The drawing under review shows one solid part. Ordinate dimensions are in mm from its lowest x, y, z. Coordinates: 2 decimals unless noted, no trailing zeros. Order: outer loops, then holes, each group sorted by start corner. A loop starts at its lowest first (then second) coordinate and runs counter-clockwise, first axis right, second up.
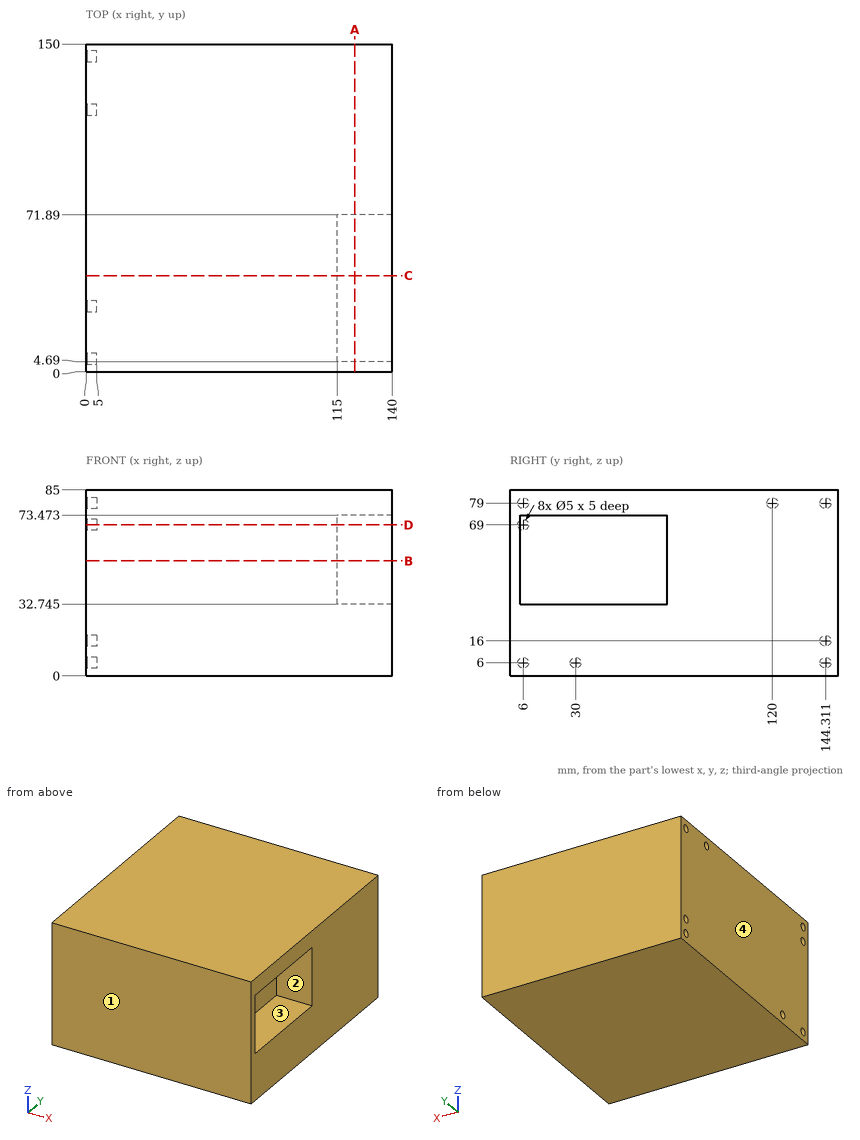
(1) Draft analysis for pull direction Y (two halves, no side actions). For the marked faces 1, 2, 3 and 4, state which applies: released by +Y, released by -Y, zero draft, split by the parting line, or undercut.
A:
face 1: released by -Y
face 2: undercut
face 3: undercut
face 4: zero draft
(2) We need section A-A, the plane x = 123. Write out the cut boundary in (y, z) (1 decimal).
A:
outline: (0, 0) - (150, 0) - (150, 85) - (0, 85) - close; hole (4.7, 32.7) - (71.9, 32.7) - (71.9, 73.5) - (4.7, 73.5) - close
(3) We need section D-D, the plane z = 69. Write out the cut boundary in (x, y), and give its area (3 significant figures).
A:
outline: (0, 0) - (140, 0) - (140, 4.69) - (115, 4.69) - (115, 71.89) - (140, 71.89) - (140, 150) - (0, 150) - (0, 8.5) - (5, 8.5) - (5, 3.5) - (0, 3.5) - close
area: 19,300 mm2
(4) We need section B-B, the plane z = 52.5. Write out the cut boundary in (x, y).
A:
outline: (0, 0) - (140, 0) - (140, 4.69) - (115, 4.69) - (115, 71.89) - (140, 71.89) - (140, 150) - (0, 150) - close
(5) We need section C-C, the plane y = 44. Write out the cut boundary in (x, z) (1 decimal).
A:
outline: (0, 0) - (140, 0) - (140, 32.7) - (115, 32.7) - (115, 73.5) - (140, 73.5) - (140, 85) - (0, 85) - close
(6) Wall thickness on probe 1 along Z at (x, y) = (3.9, 6); probe 2 along X at (y, z) = (55.5, 58): over which ranges is each line inside the solid? List them lowest first.
A:
probe 1: z = 0 to 3.5, 8.5 to 66.5, 71.5 to 76.5, 81.5 to 85
probe 2: x = 0 to 115
(7) For pin 1 Ø3 at (y, z) = (29, 67) entering from +X; pin 2 Ø1.5 at (y, z) = (145.5, 16) entering from -X, all flat-tipped, find the tip position at first contact; note any pin that passes through.
A:
pin 1: stops at x = 115
pin 2: stops at x = 5
